from build123d import *

# Parameters (mm, degrees)
SKETCH1_W          = 101.6
SKETCH1_H          = 101.6
SKETCH1_W_2        = 76.2
SKETCH1_H_2        = 76.2
SIDE_DEPTH         = 40
SKETCH1_8_W        = 76.2
SKETCH1_8_H        = 76.2
BOTTOM_DEPTH       = 15
HOLDER_DEPTH       = 25
FILLET1_R          = 10
FILLET2_R          = 10
FILLET3_R          = 10
FILLET4_R          = 10
SKETCH2_R          = 2.6
CUT_EXTRUDE1_DEPTH = 158.793298372
FILLET5_R          = 10
FILLET6_R          = 10
FILLET7_R          = 10
FILLET8_R          = 10


with BuildPart() as part:
    # Sketch1 → side (new body)
    with BuildSketch(Plane.XY):
        with Locations((50.8, 50.8)):
            Rectangle(SKETCH1_W, SKETCH1_H)
        with Locations((50.8, 50.8)):
            Rectangle(SKETCH1_W_2, SKETCH1_H_2, mode=Mode.SUBTRACT)
    extrude(amount=SIDE_DEPTH)

    # Sketch1_8 → bottom (add)
    with BuildSketch(Plane.XY):
        with Locations((50.8, 50.8)):
            Rectangle(SKETCH1_8_W, SKETCH1_8_H)
    extrude(amount=BOTTOM_DEPTH)

    # Sketch1_10 → holder (add)
    with BuildSketch(Plane.XY):
        with BuildLine():
            add(Edge.make_bspline(
                [(39.872931824, 101.6), (50.775448556, 126.225942053), (62.237812333, 101.6)],
                knots=[0, 0, 0, 1, 1, 1], degree=2))
            Line((39.872931824, 101.6), (46.872931824, 101.6))
            add(Edge.make_bspline(
                [(46.872931824, 101.6), (50.757022912, 111.505038694), (55.237812333, 101.6)],
                knots=[0, 0, 0, 1, 1, 1], degree=2))
            Line((55.237812333, 101.6), (62.237812333, 101.6))
        make_face()
    extrude(amount=HOLDER_DEPTH)

    # Fillet1
    fillet1_edges = [part.edges().sort_by_distance(p)[0] for p in [
        (0, 101.6, 20),
    ]]
    fillet(fillet1_edges, radius=FILLET1_R)

    # Fillet2
    fillet2_edges = [part.edges().sort_by_distance(p)[0] for p in [
        (0, 0, 20),
    ]]
    fillet(fillet2_edges, radius=FILLET2_R)

    # Fillet3
    fillet3_edges = [part.edges().sort_by_distance(p)[0] for p in [
        (101.6, 0, 20),
    ]]
    fillet(fillet3_edges, radius=FILLET3_R)

    # Fillet4
    fillet4_edges = [part.edges().sort_by_distance(p)[0] for p in [
        (101.6, 101.6, 20),
    ]]
    fillet(fillet4_edges, radius=FILLET4_R)

    # Sketch2 → Cut-Extrude1 (cut, through all)
    with BuildSketch(Plane(origin=(101.6, 0, 0), x_dir=(0, 0, -1), z_dir=(1, 0, 0))):
        with Locations((-11, 79.49634719)):
            Circle(SKETCH2_R)
        with Locations((-11, 20.478079238)):
            Circle(SKETCH2_R)
    extrude(amount=-CUT_EXTRUDE1_DEPTH, mode=Mode.SUBTRACT)

    # Fillet5
    fillet5_edges = [part.edges().sort_by_distance(p)[0] for p in [
        (12.7, 88.9, 27.5),
    ]]
    fillet(fillet5_edges, radius=FILLET5_R)

    # Fillet6
    fillet6_edges = [part.edges().sort_by_distance(p)[0] for p in [
        (88.9, 88.9, 27.5),
    ]]
    fillet(fillet6_edges, radius=FILLET6_R)

    # Fillet7
    fillet7_edges = [part.edges().sort_by_distance(p)[0] for p in [
        (12.7, 12.7, 27.5),
    ]]
    fillet(fillet7_edges, radius=FILLET7_R)

    # Fillet8
    fillet8_edges = [part.edges().sort_by_distance(p)[0] for p in [
        (88.9, 12.7, 27.5),
    ]]
    fillet(fillet8_edges, radius=FILLET8_R)


solid = part.part
Check sheet for the modelled part. Datum: model origin and axes. Units: mm. A direction names the side the tool comes from. Round coordinates to 2 decimals unless told otherwise and drop trailing zeros. Order: outer loops, then holes, each group sorted by start corner. A loop starts at its lowest first (then second) coordinate and runs counter-clockwise, first axis right, second up.
(1) Scan lines: probe 1 along Y at (x, z) = (73, 11); probe 2 along Y at (x, z) = (51, 20.5); probe 3 along Y at (x, z) = (52.5, 35). Record each from-to range of solid material in increasing order.
(2) Cross-section at D-D, the plane z = 27. Enter the section's corners in (x, y).
(3) Go/stop test with flat-tipped pins: P1, Ø12, axis at x = 20.5, y = 73, coming from the +Z side; P2, Ø3.5, axis at x = 47.5, y = 109, coming from the +Z side; P3, Ø6, axis at x = 66.5, z = 9, coming from the +Y side. Record where each tip stops, or that it passes through.
(4) Cross-section at C-C, the plane y = 48.5. Enter the section's corners in (x, z), and give its area (3 significant figures).
(5) Cross-section at A-A, the plane z = 11. State how many separate pieces and enclosed holes the cut face has, and give its area (3 significant figures).
(6) Draft check along Z on faces 1 (the cylindrical face through (51.511, 81.689, 9.602)), 2 (the flat face through (12.7, 50, 27)), 3 (the flat face through (95, 52, 40)). Enter one of: pulls with the +Z half, pulls with the -Z half, needs draft (parallel to the pull), parting line crosses it, or undercut.
(7) Access from +Z, -Z, +X, -X, +Y, -Y to the whole of each face (thin tool, end or side, straight path). Record for faces 4 (the flat face through (51, 108, 25)), 5 (the flat face through (50, 51, 15)), 6 (the cylindrical face through (98.75, 98.59, 20.28)).
(8) Cross-section at B-B, the plane x = 15. Enter the section's corners in (y, z).
Check sheet entries:
1. probe 1: y = 0 to 17.88, 23.08 to 76.9, 82.1 to 101.6
1. probe 2: y = 0 to 12.7, 88.9 to 101.6, 106.55 to 113.91
1. probe 3: y = 0 to 12.7, 88.9 to 101.6
2. outline: (0, 10) arc R10 ccw to (10, 0) - (91.6, 0) arc R10 ccw to (101.6, 10) - (101.6, 91.6) arc R10 ccw to (91.6, 101.6) - (10, 101.6) arc R10 ccw to (0, 91.6) - close; hole (12.7, 22.7) arc R10 ccw to (22.7, 12.7) - (78.9, 12.7) arc R10 ccw to (88.9, 22.7) - (88.9, 78.9) arc R10 ccw to (78.9, 88.9) - (22.7, 88.9) arc R10 ccw to (12.7, 78.9) - close
3. P1: stops at z = 15
3. P2: stops at z = 25
3. P3: stops at y = 101.6
4. outline: (0, 0) - (101.6, 0) - (101.6, 40) - (88.9, 40) - (88.9, 15) - (12.7, 15) - (12.7, 40) - (0, 40) - close
4. area: 2,160 mm2
5. separate pieces: 3
5. enclosed holes: 1
5. area: 9,340 mm2
6. face 1: undercut
6. face 2: needs draft
6. face 3: pulls with the +Z half
7. face 4: +Z, +X, -X, +Y
7. face 5: +Z
7. face 6: +Z, -Z, +X, +Y
8. outline: (0, 0) - (101.6, 0) - (101.6, 40) - (85.28, 40) - (85.28, 15) - (16.32, 15) - (16.32, 40) - (0, 40) - close; hole circle Ø5.2 at (20.48, 11); hole circle Ø5.2 at (79.5, 11)
